Source: CAD feature listing. Evaluate the final solid. Frame: model axes, mm. A direction names the side the tool comes from. Give positions to 0.01 mm unless a question says otherwise; leave off trailing zeros. Order: outer loops, then holes, each group sorted by start corner. A loop starts at its lowest first (then second) coordinate and runs counter-clockwise, first axis right, second up.
1) First-contact query: P1, Ø3.5, axis at y = 7, z = 1, coming from the -X side (3 decimals); P2, Ø2, axis at x = 23, z = -1.5, coming from the +Y side; P3, Ø4.5, axis at x = 24.5, y = 28.9, coming from the +Z side; P4, Ø6.5, axis at x = -14.5, y = 59.1, coming from the -Z side. Flat tips, straight axial feed; report the tip coordinate or a pass-through.
2) Draft query along Z for faces 5 (the face through (0, 45, -6)), 6 (the face through (-23, 33, -2)), 7 (the face through (-9.049, -10.001, 0.444)), 8 (the face through (0, 59, -1)). Return one class per face: released by +Z, released by -Z, zero draft, split by the parting line, or undercut.
3) Material intervals for line 1 (Y direction, x = -7, z = -2.65); line 2 (Y direction, x = 1, z = -4.5); line 3 (Z direction, x = 7, y = -8), sorted ascending.
4) Section B-B, the plane x = -7. Return loops of the section in (y, z).
5) Section C-C, the plane z = -4. Give the number of separate pieces and of enclosed holes in the cut face, plus the area to 3 significant figures.
6) Section D-D, the plane y = 78.1. Return loops of the section in (x, z).
7) Section A-A, the plane y = -8. Return loops of the section in (x, z) (3 decimals), plus the area to 3 significant figures.
8) Access query for faces 1 (the face through (3.1, 18.5, -1.6)), 2 (the face through (23, 33, -2)), 3 (the face through (0, 44.5, -3)), 4 (the face through (-9.049, 10.001, -0.444)). Directions: +Z, -Z, +X, -X, +Y, -Y. A direction counts if a zero-diameter tool reaches every point of the face in a straight line with its end or side. Return the directions, or none.
```python
from build123d import *

# Parameters (mm, degrees)
SKETCH2_R           = 2.05
BOSS_EXTRUDE1_DEPTH = 30
CUT_EXTRUDE1_START  = -12.5
SKETCH3_W           = 9.2
SKETCH3_H           = 15
SKETCH3_W_2         = 33.25
CUT_EXTRUDE1_DEPTH  = 32.5
CHAMFER1_SIZE       = 3
CHAMFER2_SIZE       = 7
SKETCH4_R           = 2.05
SKETCH4_W           = 21
SKETCH4_H           = 41
CUT_EXTRUDE2_DEPTH  = 30
SKETCH5_R           = 2.1
SKETCH5_R_2         = 1.6
CUT_EXTRUDE3_DEPTH  = 10
CUT_EXTRUDE4_DEPTH  = 10
CUT_EXTRUDE6_START  = -1
SKETCH8_W           = 2
SKETCH8_H           = 52
CUT_EXTRUDE6_DEPTH  = 2


with BuildPart() as part:
    # Sketch2 → Boss-Extrude1 (new, symmetric)
    with BuildSketch(Plane.YZ):
        Polygon((-12.5, 6), (12.5, 6), (22.5, -1), (82.5, -1), (82.5, -6), (12.5, -6), (-12.5, -6), align=None)
        with Locations(Location((-8, 0, 0), (0, 0, 270))):
            Circle(SKETCH2_R, mode=Mode.SUBTRACT)
        with Locations(Location((8, 0, 0), (0, 0, 90))):
            Circle(SKETCH2_R, mode=Mode.SUBTRACT)
    extrude(amount=BOSS_EXTRUDE1_DEPTH, both=True)

    # Sketch3 → Cut-Extrude1 (cut)
    with BuildSketch(Plane(origin=(0, 0, 0), x_dir=(-1, 0, 0), z_dir=(0, 1, 0)).offset(CUT_EXTRUDE1_START)):
        Rectangle(SKETCH3_W, SKETCH3_H)
        with Locations((-30, 0)):
            Rectangle(SKETCH3_W_2, SKETCH3_H)
        with Locations((30, 0)):
            Rectangle(SKETCH3_W_2, SKETCH3_H)
    extrude(amount=CUT_EXTRUDE1_DEPTH, mode=Mode.SUBTRACT)

    # Chamfer1
    chamfer1_edges = [part.edges().sort_by_distance(p)[0] for p in [
        (-4.6, 20, -2.625),
        (4.6, 20, -2.625),
    ]]
    chamfer(chamfer1_edges, length=CHAMFER1_SIZE)

    # Chamfer2
    chamfer2_edges = [part.edges().sort_by_distance(p)[0] for p in [
        (-13.375, 20, -2.625),
        (13.375, 20, -2.625),
    ]]
    chamfer(chamfer2_edges, length=CHAMFER2_SIZE)

    # Sketch4 → Cut-Extrude2 (cut)
    with BuildSketch(Plane(origin=(0, 0, 0), x_dir=(0, 1, 0), z_dir=(0, 0, 1))):
        with Locations(Location((39.1, 24.5, 0), (0, 0, 270))):
            Circle(SKETCH4_R)
        with Locations(Location((28.9, 24.5, 0), (0, 0, 270))):
            Circle(SKETCH4_R)
        with Locations(Location((28.9, -24.5, 0), (0, 0, 270))):
            Circle(SKETCH4_R)
        with Locations(Location((39.1, -24.5, 0), (0, 0, 270))):
            Circle(SKETCH4_R)
        with Locations((34, 0)):
            Rectangle(SKETCH4_W, SKETCH4_H)
    extrude(amount=-CUT_EXTRUDE2_DEPTH, mode=Mode.SUBTRACT)

    # Sketch5 → Cut-Extrude3 (cut)
    with BuildSketch(Plane(origin=(0, 0, 0), x_dir=(0, 1, 0), z_dir=(0, 0, 1))):
        with Locations(Location((59.1, 14.5, 0), (0, 0, 270))):
            Circle(SKETCH5_R)
        with Locations(Location((59.1, -14.5, 0), (0, 0, 270))):
            Circle(SKETCH5_R)
        with Locations(Location((78.1, 7, 0), (0, 0, 270))):
            Circle(SKETCH5_R_2)
        with Locations(Location((78.1, -7, 0), (0, 0, 270))):
            Circle(SKETCH5_R_2)
    extrude(amount=-CUT_EXTRUDE3_DEPTH, mode=Mode.SUBTRACT)

    # Sketch6 → Cut-Extrude4 (cut)
    with BuildSketch(Plane(origin=(0, 0, 0), x_dir=(0, 1, 0), z_dir=(0, 0, 1))):
        Polygon((52.5, 30), (82.5, 12.679491924), (82.5, -12.679491924), (52.5, -30), (52.5, -35), (87.5, -35), (87.5, 35), (52.5, 35), align=None)
    extrude(amount=-CUT_EXTRUDE4_DEPTH, mode=Mode.SUBTRACT)

    # Sketch8 → Cut-Extrude6 (cut)
    with BuildSketch(Plane(origin=(0, 0, 0), x_dir=(0, 1, 0), z_dir=(0, 0, 1)).offset(CUT_EXTRUDE6_START)):
        with Locations((34, 0)):
            Rectangle(SKETCH8_W, SKETCH8_H)
    extrude(amount=-CUT_EXTRUDE6_DEPTH, mode=Mode.SUBTRACT)


solid = part.part
```
From the geometry:
1. P1: stops at x = -13.375
1. P2: stops at y = 66.36
1. P3: stops at z = -1
1. P4: stops at z = -6
2. face 5: released by -Z
2. face 6: zero draft
2. face 7: undercut
2. face 8: released by +Z
3. line 1: y = -12.5 to 23.5, 44.5 to 76.5, 79.7 to 82.5
3. line 2: y = 20 to 23.5, 44.5 to 82.5
3. line 3: z = -6 to -2.05, 2.05 to 6
4. outline: (-12.5, -6) - (23.5, -6) - (23.5, -1) - (22.5, -1) - (12.5, 6) - (-12.5, 6) - close; (44.5, -6) - (76.5, -6) - (76.5, -1) - (44.5, -1) - close; (79.7, -6) - (82.5, -6) - (82.5, -1) - (79.7, -1) - close; hole circle Ø4.1 at (-8, 0); hole circle Ø4.1 at (8, 0)
5. separate pieces: 1
5. enclosed holes: 9
5. area: 2,900 mm2
6. outline: (-15.22, -6) - (-8.6, -6) - (-8.6, -1) - (-15.22, -1) - close; (-5.4, -6) - (5.4, -6) - (5.4, -1) - (-5.4, -1) - close; (8.6, -6) - (15.22, -6) - (15.22, -1) - (8.6, -1) - close
7. outline: (-13.375, -6) - (-4.6, -6) - (-4.6, -2.05) - (-13.375, -2.05) - close; (-13.375, 2.05) - (-4.6, 2.05) - (-4.6, 6) - (-13.375, 6) - close; (4.6, -6) - (13.375, -6) - (13.375, -2.05) - (4.6, -2.05) - close; (4.6, 2.05) - (13.375, 2.05) - (13.375, 6) - (4.6, 6) - close
7. area: 139 mm2
8. face 1: +Z, -Z, -Y
8. face 2: +Z
8. face 3: +Z, -Z
8. face 4: +X, -X
